Answer from the drawing. Dimensions are ordinates in mm from the lowest x, y and z of the part. Give positions to 0.01 mm unless a question says otherwise; leave off trailing zeros. Loops run counter-clockwise (first coordinate to the right, second up) from the corner with the lowest first, then second, coordinate; pieces in that order, holes last. Notation, with made-up numbers: (-22, 63) - (-2, 63) arc R30 cw to (-2, 99) - close; hole circle Ø8 at (35.25, 46.5). An arc over 180 degrees is marked (long way). Put each result on its own line as item: value. Start each with the question number.
1. Consider L1, parallel to Y at x = 115, z = 11.25; L2, parallel to Y at x = 270, z = 12.25; L3, parallel to Y at x = 123, z = 15.25. Determine where each line is inside the solid, lowest interval first. Write a range as from..to.
2. A cutting plane is placed at B-B, the plane y = 145. Determine the outline of the cut face in (x, z).
3. Given pin 1 Ø2 at (y, z) = (175.5, 7) entering from +X; pin 2 Ø18.5 at (x, y) = (305, 145) entering from +Z; pin 3 Ø5 at (y, z) = (282.5, 8) entering from -X, each flat-ended and moving along its own axis, determine where each tip first touches the part or whether it passes through.
4. A cutting plane is placed at C-C, the plane x = 370. Determine the outline of the cut face in (y, z), plus the area to 3 significant figures.
5. A cutting plane is placed at D-D, the plane z = 3.5. Count the separate pieces of the cut face and the enclosed holes in it, plus the area to 3 significant figures.
6. A cutting plane is placed at A-A, the plane x = 115. Determine the outline of the cut face in (y, z).
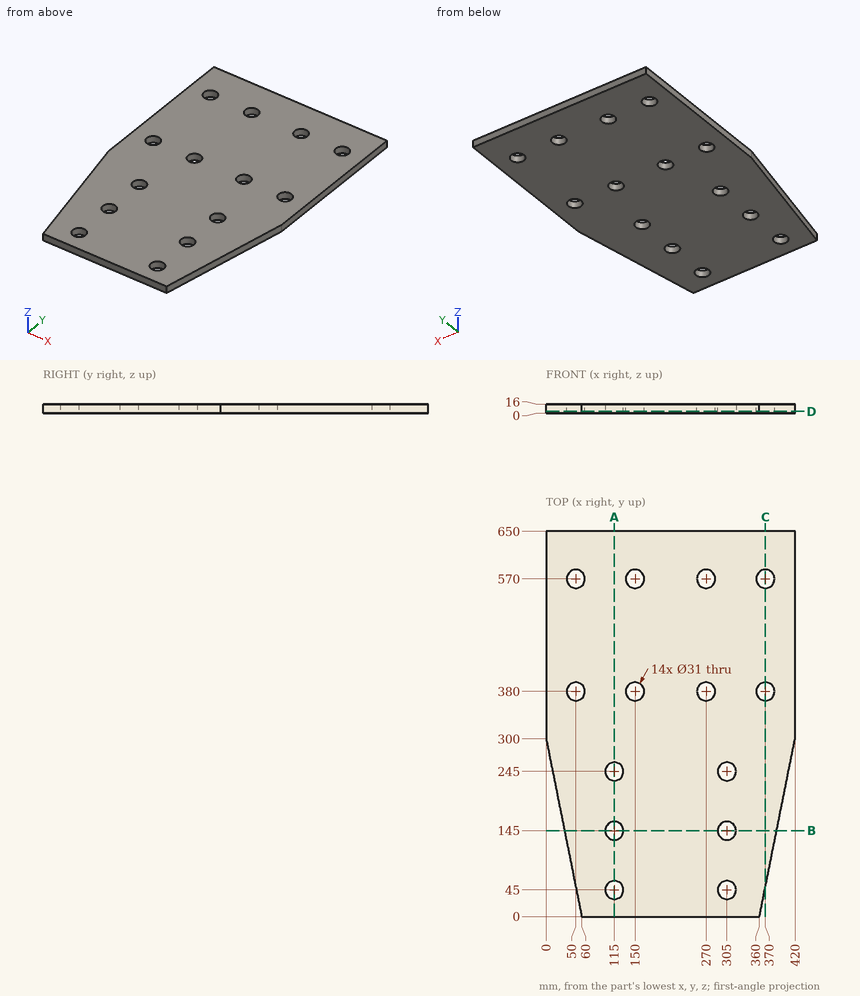
Return value:
1. L1: y = 0..29.5, 60.5..129.5, 160.5..229.5, 260.5..650
1. L2: y = 0..364.5, 395.5..554.5, 585.5..650
1. L3: y = 0..31.72, 58.28..131.72, 158.28..231.72, 258.28..650
2. outline: (31, 0) - (99.5, 0) - (99.5, 16) - (31, 16) - close; (130.5, 0) - (289.5, 0) - (289.5, 16) - (130.5, 16) - close; (320.5, 0) - (389, 0) - (389, 16) - (320.5, 16) - close
3. pin 1: stops at x = 395.3
3. pin 2: passes through
3. pin 3: stops at x = 3
4. outline: (50, 0) - (364.5, 0) - (364.5, 16) - (50, 16) - close; (395.5, 0) - (554.5, 0) - (554.5, 16) - (395.5, 16) - close; (585.5, 0) - (650, 0) - (650, 16) - (585.5, 16) - close
4. area: 8,610 mm2
5. separate pieces: 1
5. enclosed holes: 14
5. area: 244,000 mm2
6. outline: (0, 0) - (29.5, 0) - (29.5, 16) - (0, 16) - close; (60.5, 0) - (129.5, 0) - (129.5, 16) - (60.5, 16) - close; (160.5, 0) - (229.5, 0) - (229.5, 16) - (160.5, 16) - close; (260.5, 0) - (650, 0) - (650, 16) - (260.5, 16) - close
